Verification items for the finished model (mm, model axes). A direction names the side the tool comes from. Coordinates: 2 decimals unless noted, no trailing zeros. Order: outer loops, then holes, each group sorted by start corner. A loop starts at its lowest first (then second) coordinate and runs counter-clockwise, first axis right, second up. Notation, with made-up numbers: (19, 89) -> (27, 89) arc R8 ccw to (27, 96) -> close; hole circle Ø5 at (76.5, 16). An arc over 180 degrees is marked (long way). Use CSV: the item, a comma, the result in double quotes. Start each with the question number.
1) Sectioned sample at A-A on y = -2. Record the boundary of the cut face in (x, z), then the cut area to 3 significant figures.
2) Release check for a two-part mould opening along Z. For faces 1 (the flat face through (0, 15, 2)), 2 (the flat face through (6.106, -2.465, 5.832)), 3 (the flat face through (0, 0, 0)) record: released by +Z, released by -Z, zero draft, split by the parting line, or undercut.
3) Tool access check on faces 4 (the cylindrical face through (4.65, -2.54, 8.44)), 5 (the flat face through (3, -5, 9)), 6 (the flat face through (3, 0, 9)). Record the directions out of +Z, -Z, +X, -X, +Y, -Y that give a thin tool (end or side, any length) a straight path to the whole face; none if there is none.
4) Go/stop test with flat-tipped pins: pin 1 (4.5 mm diameter, centred on x = 0, z = 11, fed in from +Y); pin 2 (1.5 mm diameter, centred on y = -2.5, z = 11.5, fed in from -X); pin 3 (4.5 mm diameter, centred on x = 5, z = 10, fed in from -Y). Record where each tip stops, or that it passes through.
5) Scan lines: line 1 along Z through (x, y) = (5.5, 1); line 2 along Z through (x, y) = (-3.5, -3); line 3 along Y through (x, z) = (4.25, 13.5). Record each from-to range of solid material in increasing order.
6) Sectioned sample at B-B on y = 12. Record the boundary of the cut face in (x, z).
7) Sectioned sample at D-D on x = -2.5. Record the boundary of the cut face in (y, z), then the cut area to 3 significant figures.
from build123d import *

# Parameters (mm, degrees)
F0_W     = 30
F0_H     = 30
F1_DEPTH = 5
F3_DEPTH = 5
F4_R     = 1.6
F5_DEPTH = 20.001


with BuildPart() as f1:
    # F0 (on Top) → F1 (new body)
    with BuildSketch(Plane.XY):
        Rectangle(F0_W, F0_H)
    extrude(amount=F1_DEPTH)

    # F2 (on Front) → F3 (join)
    with BuildSketch(Plane.XZ):
        with BuildLine():
            Line((2.788165, 13.332835), (7.243725, 6.68855))
            ThreePointArc((7.243725, 6.68855), (8.533759, 8.12582), (9, 10))
            ThreePointArc((9, 10), (6.891119, 13.524723), (2.788165, 13.332835))
        make_face()
        with BuildLine():
            Line((5, 10), (5, 6))
            ThreePointArc((5, 6), (6.173499, 6.17601), (7.243725, 6.68855))
            Line((7.243725, 6.68855), (2.788165, 13.332835))
            Line((2.788165, 13.332835), (1.525476, 11.981839))
            ThreePointArc((1.525476, 11.981839), (1.1336, 11.02516), (1, 10))
            Line((1, 10), (5, 10))
        make_face()
        with BuildLine():
            ThreePointArc((1, 10), (2.171573, 7.171573), (5, 6))
            Line((5, 6), (5, 10))
            Line((5, 10), (1, 10))
        make_face()
        with BuildLine():
            Line((-3.147079, 5), (0, 5))
            Line((0, 5), (0, 10))
            Line((0, 10), (1, 10))
            ThreePointArc((1, 10), (1.1336, 11.02516), (1.525476, 11.981839))
            Line((1.525476, 11.981839), (-5, 5))
            Line((-5, 5), (-3.147079, 5))
        make_face()
        with BuildLine():
            Line((0, 10), (0, 5))
            Line((0, 5), (5, 5))
            Line((5, 5), (5, 6))
            ThreePointArc((5, 6), (2.171573, 7.171573), (1, 10))
            Line((1, 10), (0, 10))
        make_face()
        with BuildLine():
            Line((5, 6), (5, 5))
            Line((5, 5), (7.243725, 6.68855))
            ThreePointArc((7.243725, 6.68855), (6.173499, 6.17601), (5, 6))
        make_face()
    extrude(amount=F3_DEPTH)

    # F4 (on face) → F5 (cut, through all)
    with BuildSketch(Plane.XZ.offset(5)):
        with Locations((5, 10)):
            Circle(F4_R)
    extrude(amount=-F5_DEPTH, mode=Mode.SUBTRACT)


solid = f1.part
Answers follow:
1,outline,"(-15, 0) -> (15, 0) -> (15, 5) -> (5, 5) -> (7.24, 6.69) arc R4 ccw to (9, 10) arc R4 ccw to (2.79, 13.33) -> (-5, 5) -> (-15, 5) -> close; hole circle Ø3.2 at (5, 10)"
1,area,"220 mm²"
2,face 1,"zero draft"
2,face 2,"undercut"
2,face 3,"released by -Z"
3,face 4,"+Y, -Y"
3,face 5,"+Z, +X, -X, -Y"
3,face 6,"+Z, +X, -X, +Y"
4,pin 1,"stops at y = 0"
4,pin 2,"stops at x = 0.37"
4,pin 3,"stops at y = -5"
5,line 1,"z = 0 to 5"
5,line 2,"z = 0 to 6.6"
5,line 3,"y = -5 to 0"
6,outline,"(-15, 0) -> (15, 0) -> (15, 5) -> (-15, 5) -> close"
7,outline,"(-15, 0) -> (15, 0) -> (15, 5) -> (0, 5) -> (0, 7.67) -> (-5, 7.67) -> (-5, 5) -> (-15, 5) -> close"
7,area,"163 mm²"
